from build123d import *

# Parameters (mm, degrees)
EXTRUDE_1_DEPTH          = 16
CUT_EXTRUDE_1_DEPTH      = 27.111454755
CUT_EXTRUDE_1_DEPTH_BACK = 27.111454755
SKETCH_2_R               = 1.55


with BuildPart() as part:
    # ｽｹｯﾁ1 → ﾎﾞｽ - 押し出し1 (new body)
    with BuildSketch(Plane(origin=(0, 0, 0), x_dir=(1, 0, 0), z_dir=(0, 1, 0))):
        with BuildLine():
            ThreePointArc((-1.944631198, -5.764737827), (-2.486563076, -4.953679455), (-2.676864245, -3.996970874))
            Line((-2.676864245, -3.996970874), (-2.676864245, 17.239005736))
            Line((-2.676864245, 17.239005736), (-2.676864245, 18.599064096))
            Line((-2.676864245, 18.599064096), (-1.303885205, 19.972043135))
            Line((-1.303885205, 19.972043135), (0.056173154, 19.972043135))
            Line((0.056173154, 19.972043135), (1.312120474, 19.972043135))
            Line((1.312120474, 19.972043135), (1.312120474, 16.99686443))
            Line((1.312120474, 16.99686443), (1.936941769, 16.372043135))
            Line((1.936941769, 16.372043135), (2.512120474, 16.372043135))
            Line((2.512120474, 16.372043135), (2.512120474, 8.472043135))
            Line((2.512120474, 8.472043135), (1.676155012, 8.472043135))
            Line((1.676155012, 8.472043135), (1.312120474, 8.108008597))
            Line((1.312120474, 8.108008597), (1.323135755, -1.674937608))
            Line((1.323135755, -1.674937608), (1.676155012, -2.027956865))
            Line((1.676155012, -2.027956865), (3.323135755, -2.027956865))
            Line((3.323135755, -2.027956865), (3.323135755, -8.027956865))
            Line((3.323135755, -8.027956865), (1.354121746, -8.027956865))
            ThreePointArc((1.354121746, -8.027956865), (0.397413165, -7.837655696), (-0.413645207, -7.295723818))
            Line((-0.413645207, -7.295723818), (-1.944631198, -5.764737827))
        make_face()
    extrude(amount=EXTRUDE_1_DEPTH)

    # ｽｹｯﾁ2 → ｶｯﾄ - 押し出し1 (cut, two sides: drawn at the far end of the back side and taken through both)
    with BuildSketch(Plane(origin=(2.512120474, 0, 0), x_dir=(0, 0, -1), z_dir=(1, 0, 0)).offset(-CUT_EXTRUDE_1_DEPTH_BACK)):
        with Locations((12.422043135, 8)):
            Circle(SKETCH_2_R)
        with Locations((-5.027956865, 8)):
            Circle(SKETCH_2_R)
    extrude(amount=CUT_EXTRUDE_1_DEPTH + CUT_EXTRUDE_1_DEPTH_BACK, mode=Mode.SUBTRACT)


solid = part.part
Build history of the part. All positions in model axes, mm. A direction names the side the tool comes from. Coordinates: 2 decimals unless noted, no trailing zeros. Write each loop counter-clockwise with the first axis right and the second up, starting at its lowest first coordinate (ties: lowest second). Pieces come first, ordered by that corner, then holes. Notation, with made-up numbers: (64.5, 17) -> (77.5, 17) arc R10 ccw to (77.5, 25) -> close; hole circle Ø3 at (39, 43). An arc over 180 degrees is marked (long way). Use CSV: the item, a comma, the result in double quotes. Start each with the question number.
Q1. Flat gauge pins, fed straight in: pin 1 Ø2.5 at (y, z) = (11, -11) entering from +X; pin 2 Ø0.5 at (x, y) = (2.5, 9) entering from -Z; pin 3 Ø0.6 at (x, y) = (2, 8) entering from -Z. Where does each tip first touch, or does it go through?
Q2. Cut at D-D, the plane z = -5.25. List the corners of the cut face in (x, y).
Q3. 3-axis set-ups, long thin cutter, end or side, ignore diameter. For faces 4 (the flat face through (2, 8, 2.028)), 5 (the flat face through (-2, 7.888, -19.276)), 6 (the flat face through (1.312, 8, -19)): which of +Z, -Z, +X, -X, +Y, -Y reach the whole face in a straight line?
Q4. Pull direction Y, two halves, no side cores. Call faces 1 (the cylindrical face through (-0.12, 7.06, -11.19)), 2 (the flat face through (0, 16, -6)), 3 (the flat face through (2.512, 7.9, -10.7)): released by +Y, released by -Y, zero draft, split by the parting line, or undercut.
Q5. Cut at B-B, the plane y = 11. List the corners of the cut face in (x, z), then the cut area to 3 significant figures.
Q6. Cut at C-C, the plane x = 0.75. List the corners of the cut face in (y, z).
Q7. Cut at A-A, the plane y = 8. List the corners of the cut face in (x, z), then the cut area to 3 significant figures.
Q8. Drill centre lines: probe 1 along Z at (x, y) = (1.4, 8); probe 2 along Z at (x, y) = (1, 8); probe 3 along X at (y, z) = (2, -2.25). Where is each one in solid material? Low to high.
Checked values:
1,pin 1,"stops at x = 2.51"
1,pin 2,"stops at z = -16.37"
1,pin 3,"stops at z = -16.61"
2,outline,"(-2.68, 0) -> (1.32, 0) -> (1.32, 16) -> (-2.68, 16) -> close"
3,face 4,"+X, +Y, -Y"
3,face 5,"-Z, -X, +Y, -Y"
3,face 6,"-Z, +X, +Y, -Y"
4,face 1,"undercut"
4,face 2,"released by +Y"
4,face 3,"zero draft"
5,outline,"(-2.68, -18.6) -> (-1.3, -19.97) -> (1.31, -19.97) -> (1.31, -17) -> (1.94, -16.37) -> (2.51, -16.37) -> (2.51, -8.47) -> (1.68, -8.47) -> (1.31, -8.11) -> (1.32, 1.67) -> (1.68, 2.03) -> (3.32, 2.03) -> (3.32, 8.03) -> (1.35, 8.03) arc R2.5 ccw to (-0.41, 7.3) -> (-1.94, 5.76) arc R2.5 ccw to (-2.68, 4) -> close"
5,area,"128 mm²"
6,outline,"(0, -19.97) -> (16, -19.97) -> (16, 7.95) -> (0, 7.95) -> close; hole circle Ø3.1 at (8, -12.42); hole circle Ø3.1 at (8, 5.03)"
7,outline,"(-2.68, -18.6) -> (-1.3, -19.97) -> (1.31, -19.97) -> (1.31, -17) -> (1.94, -16.37) -> (2.51, -16.37) -> (2.51, -13.97) -> (-2.68, -13.97) -> close; (-2.68, -10.87) -> (2.51, -10.87) -> (2.51, -8.47) -> (1.68, -8.47) -> (1.31, -8.11) -> (1.32, 1.67) -> (1.68, 2.03) -> (3.32, 2.03) -> (3.32, 3.48) -> (-2.68, 3.48) -> close; (-1.13, 6.58) -> (3.32, 6.58) -> (3.32, 8.03) -> (1.35, 8.03) arc R2.5 ccw to (-0.41, 7.3) -> close"
7,area,"94.6 mm²"
8,probe 1,"z = -16.91 to -13.97, -10.87 to -8.2, 1.75 to 3.48, 6.58 to 8.03"
8,probe 2,"z = -19.97 to -13.97, -10.87 to 3.48, 6.58 to 8"
8,probe 3,"x = -2.68 to 1.32"
